```python
from build123d import *

# Parameters (mm, degrees)
SALIENTE_EXTRUIR1_DEPTH = 11.5
CROQUIS2_R              = 4.71
SALIENTE_EXTRUIR2_DEPTH = 47.82
CROQUIS3_R              = 2.5
CORTAR_EXTRUIR1_DEPTH   = 10


with BuildPart() as part:
    # Croquis1 → Saliente-Extruir1 (new body)
    with BuildSketch(Plane.XY):
        Polygon((0, 7.216878365), (-6.25, 3.608439182), (-6.25, -3.608439182), (0, -7.216878365), (6.25, -3.608439182), (6.25, 3.608439182), align=None)
    extrude(amount=SALIENTE_EXTRUIR1_DEPTH)

    # Croquis2 → Saliente-Extruir2 (add)
    with BuildSketch(Plane.XY.offset(11.5)):
        Circle(CROQUIS2_R)
    extrude(amount=SALIENTE_EXTRUIR2_DEPTH)

    # Croquis3 → Cortar-Extruir1 (cut)
    with BuildSketch(Plane.XY.offset(59.32)):
        Circle(CROQUIS3_R)
    extrude(amount=-CORTAR_EXTRUIR1_DEPTH, mode=Mode.SUBTRACT)


solid = part.part
```
Here's how the part is built. I have some questions about the finished solid (model axes, mm). A direction names the side the tool comes from. Coordinates: 2 decimals unless noted, no trailing zeros. Order: outer loops, then holes, each group sorted by start corner. A loop starts at its lowest first (then second) coordinate and runs counter-clockwise, first axis right, second up.
Item 1: I'm going to push flat-ended pins straight in: pin 1 Ø1.5 at (x, y) = (-0.5, -0.5) entering from +Z; pin 2 Ø4 at (y, z) = (3.5, 27) entering from -X; pin 3 Ø5 at (y, z) = (-4, 33.5) entering from +X. Where does each tip first touch, or does it pass through?
Response values:
pin 1: stops at z = 49.32
pin 2: stops at x = -4.46
pin 3: stops at x = 4.46
Item 2: Which directions (+Z, -Z, +X, -X, +Y, -Y) give clear straight access to the entire face, cutting with the end or side of a thin tool? Please do faces 1 (the face through (0, 0, 0)), 2 (the face through (-0.54, -2.44, 54.39)).
Response values:
face 1: -Z, +X, -X, +Y, -Y
face 2: +Z
Item 3: If we section it at B-B, the plane x = -1: List the corners of the cut face in (y, z) for me, then the cut area to 3 significant figures.
Response values:
outline: (-6.64, 0) - (6.64, 0) - (6.64, 11.5) - (4.6, 11.5) - (4.6, 59.32) - (2.29, 59.32) - (2.29, 49.32) - (-2.29, 49.32) - (-2.29, 59.32) - (-4.6, 59.32) - (-4.6, 11.5) - (-6.64, 11.5) - close
area: 547 mm2
Item 4: If we section it at A-A, the plane y = 0: List the corners of the cut face in (x, z) for me, then the cut area to 3 significant figures.
Response values:
outline: (-6.25, 0) - (6.25, 0) - (6.25, 11.5) - (4.71, 11.5) - (4.71, 59.32) - (2.5, 59.32) - (2.5, 49.32) - (-2.5, 49.32) - (-2.5, 59.32) - (-4.71, 59.32) - (-4.71, 11.5) - (-6.25, 11.5) - close
area: 544 mm2
Item 5: I need wall thicknesses on probe 1 along Y at (x, z) = (0, 52.5); probe 2 along Z at (x, y) = (5.25, -2); probe 3 along X at (y, z) = (-0.25, 12). Which ranges of each line are inside material? Lowest first, please.
Response values:
probe 1: y = -4.71 to -2.5, 2.5 to 4.71
probe 2: z = 0 to 11.5
probe 3: x = -4.7 to 4.7
Item 6: Thinking about a two-plate mould opening in X: for faces 3 (the face through (3.169, 5.387, 5.67)), 4 (the face through (0, 0, 49.32)), 5 (the face through (-3.08, 5.44, 5.67)), which applies, pulls with the +X half, pulls with the -X half, needs draft (parallel to the pull), parting line crosses it, or undercut?
Response values:
face 3: pulls with the +X half
face 4: undercut
face 5: pulls with the -X half
Item 7: If we section it at C-C, the plane z = 18: List the corners of the cut face in (x, y) for me.
Response values:
outline: circle Ø9.42 at (0, 0)
Item 8: If we section it at D-D, the plane z = 5: List the corners of the cut face in (x, y) for me, then the cut area to 3 significant figures.
Response values:
outline: (-6.25, -3.61) - (0, -7.22) - (6.25, -3.61) - (6.25, 3.61) - (0, 7.22) - (-6.25, 3.61) - close
area: 135 mm2
